```python
from build123d import *

# Parameters (mm, degrees)
EXTRUDE_1_DEPTH     = 8.9
CUT_EXTRUDE_START   = 163.3
SKETCH_2_R          = 0.6
SKETCH_2_RX         = 2.25
SKETCH_2_RY         = 1.9
SKETCH_2_RX_2       = 1.9
SKETCH_2_RY_2       = 0.5
CUT_EXTRUDE_5_DEPTH = 8.9
SKETCH_7_OUTSIDE_W  = 201.53
SKETCH_7_OUTSIDE_H  = 47.13
CUT_EXTRUDE_6_DEPTH = 0.5
CUT_EXTRUDE_7_DEPTH = 0.5


with BuildPart() as part:
    # 草图1 → 凸台-拉伸1 (new body)
    with BuildSketch(Plane(origin=(0, 0, 0), x_dir=(1, 0, 0), z_dir=(0, 1, 0))):
        with BuildLine():
            Line((10, 0), (153.3, 0))
            ThreePointArc((153.3, 0), (160.371067812, 2.928932188), (163.3, 10))
            Line((163.3, 10), (163.3, 67.9))
            ThreePointArc((163.3, 67.9), (160.371067812, 74.971067812), (153.3, 77.9))
            Line((153.3, 77.9), (10, 77.9))
            ThreePointArc((10, 77.9), (2.928932188, 74.971067812), (0, 67.9))
            Line((0, 67.9), (0, 10))
            ThreePointArc((0, 10), (2.928932188, 2.928932188), (10, 0))
        make_face()
    extrude(amount=EXTRUDE_1_DEPTH)

    # 草图2 → 切除-拉伸5 (cut)
    # profile 1 of 10: a face of its own
    with BuildSketch(Plane(origin=(0, 0, 0), x_dir=(0, 0, -1), z_dir=(1, 0, 0)).offset(CUT_EXTRUDE_START)):
        with Locations(Location((48.272527564, 4.45, 0), (0, 0, 180))):
            Circle(SKETCH_2_R)
    # profile 2 of 10: a face of its own
    with BuildSketch(Plane(origin=(0, 0, 0), x_dir=(0, 0, -1), z_dir=(1, 0, 0)).offset(CUT_EXTRUDE_START)):
        with Locations(Location((14.485427664, 4.45), (0, 0, 180))):
            Ellipse(SKETCH_2_RX, SKETCH_2_RY)
    # profile 3 of 10: a face of its own
    with BuildSketch(Plane(origin=(0, 0, 0), x_dir=(0, 0, -1), z_dir=(1, 0, 0)).offset(CUT_EXTRUDE_START)):
        with Locations(Location((19.399284115, 4.45), (0, 0, 90))):
            Ellipse(SKETCH_2_RX_2, SKETCH_2_RY_2)
    # profile 4 of 10: a face of its own
    with BuildSketch(Plane(origin=(0, 0, 0), x_dir=(0, 0, -1), z_dir=(1, 0, 0)).offset(CUT_EXTRUDE_START)):
        with Locations(Location((20.899284115, 4.45), (0, 0, 90))):
            Ellipse(SKETCH_2_RX_2, SKETCH_2_RY_2)
    # profile 5 of 10: a face of its own
    with BuildSketch(Plane(origin=(0, 0, 0), x_dir=(0, 0, -1), z_dir=(1, 0, 0)).offset(CUT_EXTRUDE_START)):
        with Locations(Location((22.399284115, 4.45), (0, 0, 90))):
            Ellipse(SKETCH_2_RX_2, SKETCH_2_RY_2)
    # profile 6 of 10: a face of its own
    with BuildSketch(Plane(origin=(0, 0, 0), x_dir=(0, 0, -1), z_dir=(1, 0, 0)).offset(CUT_EXTRUDE_START)):
        with Locations(Location((23.899284115, 4.45), (0, 0, 90))):
            Ellipse(SKETCH_2_RX_2, SKETCH_2_RY_2)
    # profile 7 of 10: a face of its own
    with BuildSketch(Plane(origin=(0, 0, 0), x_dir=(0, 0, -1), z_dir=(1, 0, 0)).offset(CUT_EXTRUDE_START)):
        with Locations(Location((25.399284115, 4.45), (0, 0, 90))):
            Ellipse(SKETCH_2_RX_2, SKETCH_2_RY_2)
    # profile 8 of 10: a face of its own
    with BuildSketch(Plane(origin=(0, 0, 0), x_dir=(0, 0, -1), z_dir=(1, 0, 0)).offset(CUT_EXTRUDE_START)):
        with Locations(Location((26.899284115, 4.45), (0, 0, 90))):
            Ellipse(SKETCH_2_RX_2, SKETCH_2_RY_2)
    # profile 9 of 10: a face of its own
    with BuildSketch(Plane(origin=(0, 0, 0), x_dir=(0, 0, -1), z_dir=(1, 0, 0)).offset(CUT_EXTRUDE_START)):
        with BuildLine():
            Line((41.95, 2.95), (35.95, 2.95))
            ThreePointArc((35.95, 2.95), (34.45, 4.45), (35.95, 5.95))
            Line((35.95, 5.95), (41.95, 5.95))
            ThreePointArc((41.95, 5.95), (43.45, 4.45), (41.95, 2.95))
        make_face()
    # profile 10 of 10: a face of its own
    with BuildSketch(Plane(origin=(0, 0, 0), x_dir=(0, 0, -1), z_dir=(1, 0, 0)).offset(CUT_EXTRUDE_START)):
        with BuildLine():
            Line((60.478464751, 3.2), (50.871535249, 3.2))
            ThreePointArc((50.871535249, 3.2), (49.621535249, 4.45), (50.871535249, 5.7))
            Line((50.871535249, 5.7), (60.478464751, 5.7))
            ThreePointArc((60.478464751, 5.7), (61.728464751, 4.45), (60.478464751, 3.2))
        make_face()
        with Locations(Location((50.871535249, 4.45, 0), (0, 0, 180))):
            Circle(SKETCH_2_R, mode=Mode.SUBTRACT)
    extrude(amount=-CUT_EXTRUDE_5_DEPTH, mode=Mode.SUBTRACT)

    # 草图7 outside → 切除-拉伸6 (cut)
    with BuildSketch(Plane.XY):
        with Locations((81.65, 4.45)):
            Rectangle(SKETCH_7_OUTSIDE_W, SKETCH_7_OUTSIDE_H)
        with BuildLine():
            Line((33.826473294, 3.502985919), (47.039275266, 3.502985919))
            ThreePointArc((47.039275266, 3.502985919), (47.392828657, 3.649432529), (47.539275266, 4.002985919))
            Line((47.539275266, 4.002985919), (47.539275266, 4.897014081))
            ThreePointArc((47.539275266, 4.897014081), (47.392828657, 5.250567471), (47.039275266, 5.397014081))
            Line((47.039275266, 5.397014081), (33.826473294, 5.397014081))
            ThreePointArc((33.826473294, 5.397014081), (33.472919903, 5.250567471), (33.326473294, 4.897014081))
            Line((33.326473294, 4.897014081), (33.326473294, 4.002985919))
            ThreePointArc((33.326473294, 4.002985919), (33.472919903, 3.649432529), (33.826473294, 3.502985919))
        make_face(mode=Mode.SUBTRACT)
        with BuildLine():
            Line((61.422997124, 3.502985919), (68.003158176, 3.502985919))
            ThreePointArc((68.003158176, 3.502985919), (68.356711566, 3.649432529), (68.503158176, 4.002985919))
            Line((68.503158176, 4.002985919), (68.503158176, 4.897014081))
            ThreePointArc((68.503158176, 4.897014081), (68.356711566, 5.250567471), (68.003158176, 5.397014081))
            Line((68.003158176, 5.397014081), (61.422997124, 5.397014081))
            ThreePointArc((61.422997124, 5.397014081), (61.069443733, 5.250567471), (60.922997124, 4.897014081))
            Line((60.922997124, 4.897014081), (60.922997124, 4.002985919))
            ThreePointArc((60.922997124, 4.002985919), (61.069443733, 3.649432529), (61.422997124, 3.502985919))
        make_face(mode=Mode.SUBTRACT)
    extrude(amount=-CUT_EXTRUDE_6_DEPTH, mode=Mode.SUBTRACT)

    # 草图8 → 切除-拉伸7 (cut)
    with BuildSketch(Plane.XZ):
        with BuildLine():
            Line((1.465261874, -67.9), (1.465261874, -10))
            ThreePointArc((1.465261874, -10), (3.965028796, -3.965028796), (10, -1.465261874))
            Line((10, -1.465261874), (153.3, -1.465261874))
            ThreePointArc((153.3, -1.465261874), (159.334971204, -3.965028796), (161.834738126, -10))
            Line((161.834738126, -10), (161.834738126, -67.9))
            ThreePointArc((161.834738126, -67.9), (159.334971204, -73.934971204), (153.3, -76.434738126))
            Line((153.3, -76.434738126), (10, -76.434738126))
            ThreePointArc((10, -76.434738126), (3.965028796, -73.934971204), (1.465261874, -67.9))
        make_face()
    extrude(amount=-CUT_EXTRUDE_7_DEPTH, mode=Mode.SUBTRACT)


solid = part.part
```
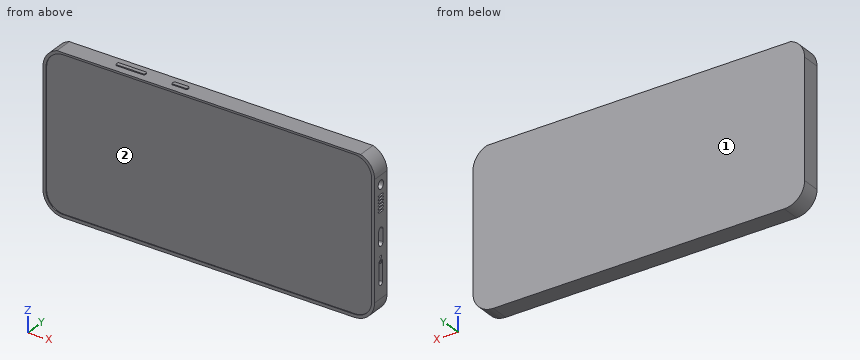
CAD build for the part. Positions are in the model's coordinates, mm. Face numbers are marked on the shaded views. Give positions to 0.01 mm unless a question says otherwise; leave off trailing zeros. Order: outer loops, then holes, each group sorted by start corner. A loop starts at its lowest first (then second) coordinate and runs counter-clockwise, first axis right, second up.
(1) Saw through at B-B, the plane x = 56.5. Give the cut face in (y, z), then the cut area to 3 significant figures.
(2) Saw through at C-C, the plane x = 37. Give the cut face in (y, z).
(3) Drill centre lines: L1, parallel to Z at x = 32.5, y = 2.75; L2, parallel to X at y = 6, z = -15; L3, parallel to Y at x = 134, z = -67. Where is each one in solid material? Low to high.
(4) Saw through at A-A, the plane z = -58.5. Give the cut face in (x, y).
(5) Flat gauge pins, fed straight in: pin 1 (7 mm diameter, centred on x = 160, z = -53.5, fed in from -Y); pin 2 (8 mm diameter, centred on x = 109, z = -50, fed in from -Y); pin 3 (0.6 mm diameter, centred on y = 4.5, z = -0.5, fed in from -X). Where does each tip first touch, or does it go through?
(6) Mould opens along Z. For the marked faces 1 and 2 say: released by +Z, released by -Z, zero draft, split by the parting line, or undercut.
(7) Saw through at D-D, the plane z = -30. Give the cut face in (x, y), then the cut area to 3 significant figures.
Results found:
1. outline: (0, -77.9) - (8.9, -77.9) - (8.9, -0.5) - (0, -0.5) - (0, -1.47) - (0.5, -1.47) - (0.5, -76.43) - (0, -76.43) - close
1. area: 651 mm2
2. outline: (0, -77.9) - (8.9, -77.9) - (8.9, -0.5) - (5.4, -0.5) - (5.4, 0) - (3.5, 0) - (3.5, -0.5) - (0, -0.5) - (0, -1.47) - (0.5, -1.47) - (0.5, -76.43) - (0, -76.43) - close
3. L1: z = -77.9 to -0.5
3. L2: x = 0 to 154.4
3. L3: y = 0.5 to 8.9
4. outline: (0, 0) - (1.47, 0) - (1.47, 0.5) - (161.83, 0.5) - (161.83, 0) - (163.3, 0) - (163.3, 3.2) - (154.4, 3.2) - (154.4, 5.7) - (163.3, 5.7) - (163.3, 8.9) - (0, 8.9) - close
5. pin 1: stops at y = 0
5. pin 2: stops at y = 0.5
5. pin 3: stops at x = 6.08
6. face 1: zero draft
6. face 2: undercut
7. outline: (0, 0) - (1.47, 0) - (1.47, 0.5) - (161.83, 0.5) - (161.83, 0) - (163.3, 0) - (163.3, 8.9) - (0, 8.9) - close
7. area: 1,370 mm2
